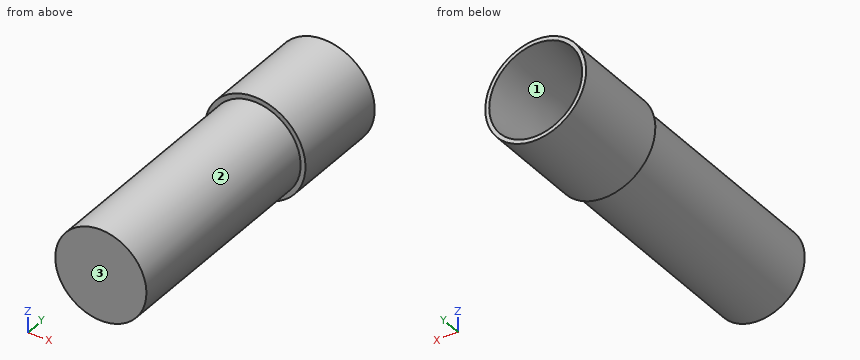
```python
from build123d import *

# Parameters (mm, degrees)
SKETCH1_R           = 12.7
BOSS_EXTRUDE1_DEPTH = 82
SKETCH2_R           = 11.7
CUT_EXTRUDE1_DEPTH  = 25.4
CUT_EXTRUDE1_DRAFT  = -5
SKETCH3_R           = 9.477787946
CUT_EXTRUDE2_DEPTH  = 53.38
SKETCH5_OUTSIDE_W   = 45.304
SKETCH5_OUTSIDE_H   = 45.304
SKETCH5_OUTSIDE_R   = 11.477787946
CUT_EXTRUDE4_DEPTH  = 60.374839676


with BuildPart() as part:
    # Sketch1 → Boss-Extrude1 (new body)
    with BuildSketch(Plane(origin=(0, 0, 0), x_dir=(1, 0, 0), z_dir=(0, 1, 0))):
        with Locations(Location((0, 0, 0), (0, 0, 270))):
            Circle(SKETCH1_R)
    extrude(amount=-BOSS_EXTRUDE1_DEPTH)


with BuildPart() as cut_extrude1_tool:
    # Sketch2 → Cut-Extrude1 (with draft: the straight prism first)
    with BuildSketch(Plane(origin=(0, 0, 0), x_dir=(1, 0, 0), z_dir=(0, 1, 0))):
        Circle(SKETCH2_R)
    extrude(amount=-CUT_EXTRUDE1_DEPTH)
    # Cut-Extrude1: the draft: its side faces are tilted about the plane it starts from
    cut_extrude1_sides = [cut_extrude1_tool.faces().sort_by_distance(p)[0] for p in [
        (-11.7, -12.7, 0),
    ]]
    draft(cut_extrude1_sides, Plane(origin=(0, 0, 0), x_dir=(1, 0, 0), z_dir=(0, 1, 0)), CUT_EXTRUDE1_DRAFT)


with BuildPart() as part_1:
    add(part.part)

    # Cut-Extrude1: cut by cut_extrude1_tool
    add(cut_extrude1_tool.part, mode=Mode.SUBTRACT)

    # Sketch3 → Cut-Extrude2 (cut)
    with BuildSketch(Plane(origin=(0, -25.4, 0), x_dir=(1, 0, 0), z_dir=(0, 1, 0))):
        with Locations(Location((0, 0, 0), (0, 0, 270))):
            Circle(SKETCH3_R)
    extrude(amount=-CUT_EXTRUDE2_DEPTH, mode=Mode.SUBTRACT)

    # Sketch5 outside → Cut-Extrude4 (cut, through all)
    with BuildSketch(Plane(origin=(0, -25.406788512, 0), x_dir=(1, 0, 0), z_dir=(0, 1, 0))):
        Rectangle(SKETCH5_OUTSIDE_W, SKETCH5_OUTSIDE_H)
        with Locations(Location((0, 0, 0), (0, 0, 270))):
            Circle(SKETCH5_OUTSIDE_R, mode=Mode.SUBTRACT)
    extrude(amount=-CUT_EXTRUDE4_DEPTH, mode=Mode.SUBTRACT)


solid = part_1.part
```
Read the model definition and answer for the solid it produces. Units are mm, in the model's axes. Face numbers are marked on the shaded views. Round coordinates to 2 decimals unless told otherwise and drop trailing zeros. Loops run counter-clockwise (first coordinate to the right, second up) from the corner with the lowest first, then second, coordinate; pieces in that order, holes last. Notation, with made-up numbers: (-38.75, 73.5) -> (12.25, 73.5) arc R11 ccw to (12.25, 88.5) -> close; hole circle Ø2 at (64.5, 89.25). An arc over 180 degrees is marked (long way). One line per item, written item: value.
1) A cutting plane is placed at C-C (y = -38.5). Determine the outline of the cut face in (x, z), and give its area (3 significant figures).
Answer list:
outline: circle Ø22.96 at (0, 0); hole circle Ø18.96 at (0, 0)
area: 132 mm²
2) Flat-ended cylindrical pins translate along their axes: P1, Ø1.5, axis at x = 6, y = -61.5, coming from the +Z side; P2, Ø5, axis at x = 9, y = -30, coming from the +Z side; P3, Ø8, axis at x = -6.5, y = -67, coming from the -Z side. Find the tip coordinate at first contact, or state that the pin passes through.
Answer list:
P1: stops at z = 10.21
P2: stops at z = 9.46
P3: stops at z = -11.2
3) A cutting plane is placed at A-A (z = 0). Determine the outline of the cut face in (x, y), and give its area (3 significant figures).
Answer list:
outline: (-12.7, -25.41) -> (-11.48, -25.41) -> (-11.48, -82) -> (11.48, -82) -> (11.48, -25.41) -> (12.7, -25.41) -> (12.7, 0) -> (11.7, 0) -> (9.48, -25.4) -> (9.48, -78.78) -> (-9.48, -78.78) -> (-9.48, -25.4) -> (-11.7, 0) -> (-12.7, 0) -> close
area: 395 mm²
4) The mould has two halves that part along X. Classify the marked faces 1, 2 and 3: pulls with the +X half, pulls with the -X half, needs draft (parallel to the pull), parting line crosses it, or undercut.
Answer list:
face 1: undercut
face 2: parting line crosses it
face 3: needs draft
5) A cutting plane is placed at B-B (x = 0). Determine the outline of the cut face in (y, z), and give its area (3 significant figures).
Answer list:
outline: (-82, -11.48) -> (-25.41, -11.48) -> (-25.41, -12.7) -> (0, -12.7) -> (0, -11.7) -> (-25.4, -9.48) -> (-78.78, -9.48) -> (-78.78, 9.48) -> (-25.4, 9.48) -> (0, 11.7) -> (0, 12.7) -> (-25.41, 12.7) -> (-25.41, 11.48) -> (-82, 11.48) -> close
area: 395 mm²
6) Consider L1, parallel to X at y = -64.5, z = 0; L2, parallel to Y at x = 1.5, z = -4; L3, parallel to Z at x = 3, y = -54.5. Determine where each line is inside the solid, lowest interval first. Write a range as [from, to].
Answer list:
L1: x = [-11.48, -9.48], [9.48, 11.48]
L2: y = [-82, -78.78]
L3: z = [-11.08, -8.99], [8.99, 11.08]
